```python
from build123d import *

# Parameters (mm, degrees)
SKETCH1_W           = 50
SKETCH1_H           = 50
BOSS_EXTRUDE1_DEPTH = 3
SKETCH3_R           = 14
SKETCH3_R_2         = 12.5
SKETCH4_R           = 2.5
CUT_EXTRUDE13_DEPTH = 3
SKETCH8_R           = 2.5
CUT_EXTRUDE20_DEPTH = 3
CUT_EXTRUDE22_DEPTH = 21
CIRPATTERN4_COUNT   = 4


with BuildPart() as part:
    # Sketch1 → Boss-Extrude1 (new body)
    with BuildSketch(Plane(origin=(0, 0, 0), x_dir=(1, 0, 0), z_dir=(0, 1, 0))):
        Rectangle(SKETCH1_W, SKETCH1_H)
    extrude(amount=BOSS_EXTRUDE1_DEPTH)

    # Sweep1: sweep along a path in Sketch2
    with BuildLine(Plane.XY) as sweep1_path:
        Line((0, 3), (25, 46.301270189))
    # Sketch3 → Sweep1 (sweep)
    with BuildSketch(Plane(origin=(0, 3, 0), x_dir=(1, 0, 0), z_dir=(0, 1, 0))):
        Circle(SKETCH3_R)
        Circle(SKETCH3_R_2, mode=Mode.SUBTRACT)
    sweep(path=sweep1_path.line)

    # Sketch4 → Cut-Extrude13 (cut)
    with BuildSketch(Plane(origin=(0, 0, 0), x_dir=(1, 0, 0), z_dir=(0, 1, 0))):
        with Locations((-20, 20)):
            Circle(SKETCH4_R)
    cut_extrude13 = extrude(amount=CUT_EXTRUDE13_DEPTH, mode=Mode.SUBTRACT)

    # Sketch8 → Cut-Extrude20 (cut)
    with BuildSketch(Plane(origin=(0, 0, 0), x_dir=(1, 0, 0), z_dir=(0, 1, 0))):
        with Locations((20, 20)):
            Circle(SKETCH8_R)
    cut_extrude20 = extrude(amount=CUT_EXTRUDE20_DEPTH, mode=Mode.SUBTRACT)

    # Mirror1: Cut-Extrude20 across plane
    add(cut_extrude20.mirror(Plane.XY), mode=Mode.SUBTRACT)

    # Mirror2: Cut-Extrude13 across plane
    add(cut_extrude13.mirror(Plane.XY), mode=Mode.SUBTRACT)

    # Sketch9 → Cut-Extrude22 (cut)
    with BuildSketch(Plane(origin=(0, 0, 0), x_dir=(1, 0, 0), z_dir=(0, 1, 0))):
        with BuildLine():
            Line((-10, 30), (10, 30))
            ThreePointArc((10, 30), (15, 25), (10, 20))
            Line((10, 20), (-10, 20))
            ThreePointArc((-10, 20), (-15, 25), (-10, 30))
        make_face()
    cut_extrude22 = extrude(amount=CUT_EXTRUDE22_DEPTH, mode=Mode.SUBTRACT)

    # CirPattern4: Cut-Extrude22 ×4 about axis
    cirpattern4_axis = Axis((0, 0, 0), (0, 1, 0))
    for i in range(1, CIRPATTERN4_COUNT):
        add(cut_extrude22.rotate(cirpattern4_axis, i * 360 / CIRPATTERN4_COUNT), mode=Mode.SUBTRACT)


solid = part.part
```
Geometry: final body of the model. Coordinates: model frame, mm. A direction names the side the tool comes from. Coordinates: 2 decimals unless noted, no trailing zeros. Write each question's results on one line, items separated by ' | '.
(1) Mould query, pull axis X, two halves, no side actions, for faces 1 (the face through (-22, 1, -14)), 2 (the face through (14, 1, -22)), 3 (the face through (22, 1, 14)). Classes: +X half, -X half, draft (parallel to the pull), parting line (faces both ways), or undercut.
Values found:
face 1: -X half | face 2: undercut | face 3: +X half
(2) First-contact query: pin 1 Ø12 at (x, y) = (-18, 7.5) entering from +Z; pin 2 Ø8 at (x, y) = (3, 34) entering from +Z; pin 3 Ø10 at (y, z) = (17.5, -9.5) entering from -X; pin 4 Ø6 at (y, z) = (16.5, 2) entering from +X. Flat tips, straight axial feed; report the tip coordinate or a pass-through.
Values found:
pin 1: stops at z = 25 | pin 2: stops at z = 9.5 | pin 3: stops at x = -6.35 | pin 4: stops at x = 20
(3) Set-up query: faces 4 (the face through (0, 1, 20)), 5 (the face through (21, 1, -13)), 6 (the face through (23.3, 21, 0)), 7 (the face through (0, 1, -20)). Return all of +Z, -Z, +X, -X, +Y, -Y with unobstructed straight access to the full face (end or side cutting, diameter ignored); none if empty.
Values found:
face 4: +Z, +Y, -Y | face 5: +X, -Y | face 6: +Z, -Z, +X, -Y | face 7: -Z, +Y, -Y
(4) Line query: line 1 (Z direction, x = 22.5, y = 42); line 2 (Y direction, x = -11, z = 16); line 3 (X direction, y = 30, z = 3). Output: solid intervals per line, ascending. Write a range as [from, to].
Values found:
line 1: z = [-14, -12.5], [12.5, 14] | line 2: y = [0, 3] | line 3: x = [1.91, 3.45], [27.72, 29.26]
